```python
from build123d import *

# Parameters (mm, degrees)
BOSS_EXTRUDE1_DEPTH = 19.05
SKETCH2_R           = 3.96875
CUT_EXTRUDE1_DEPTH  = 19.05
SKETCH3_W           = 457.2
SKETCH3_H           = 152.4
BOSS_EXTRUDE3_DEPTH = 19.05
SKETCH4_W           = 457.2
SKETCH4_H           = 152.4
CUT_EXTRUDE2_DEPTH  = 25.4
CUT_EXTRUDE3_DEPTH  = 25.4
BOSS_EXTRUDE4_DEPTH = 3.175


with BuildPart() as part:
    # Sketch1 → Boss-Extrude1 (new body)
    with BuildSketch(Plane(origin=(0, 0, 0), x_dir=(1, 0, 0), z_dir=(0, 1, 0))):
        Polygon((57.15, 19.05), (0, 19.05), (0, 0), (66.037825848, 0), (97.808358016, 38.1), (336.311308439, 38.1), (400.965853894, -12.7), (431.8, -12.7), (342.9, 57.15), (88.9, 57.15), align=None)
    extrude(amount=BOSS_EXTRUDE1_DEPTH)

    # Sketch2 → Cut-Extrude1 (cut)
    with BuildSketch(Plane.XY):
        with Locations((8.89, 9.525)):
            Circle(SKETCH2_R)
        with Locations((56.515, 9.525)):
            Circle(SKETCH2_R)
    extrude(amount=-CUT_EXTRUDE1_DEPTH, mode=Mode.SUBTRACT)

    # Sketch4 → Cut-Extrude2 (cut)
    with BuildSketch(Plane(origin=(0, 0, 0), x_dir=(1, 0, 0), z_dir=(0, 1, 0))):
        with Locations((215.9, 38.1)):
            Rectangle(SKETCH4_W, SKETCH4_H)
    extrude(amount=CUT_EXTRUDE2_DEPTH, mode=Mode.SUBTRACT)


with BuildPart() as body_2:
    # Sketch3 → Boss-Extrude3 (new body)
    with BuildSketch(Plane.XZ):
        with Locations((215.9, -38.1)):
            Rectangle(SKETCH3_W, SKETCH3_H)
        Polygon((400.965853894, 12.7), (431.8, 12.7), (342.9, -57.15), (88.9, -57.15), (57.15, -19.05), (0, -19.05), (0, 0), (66.037825848, 0), (97.808358016, -38.1), (336.311308439, -38.1), align=None, mode=Mode.SUBTRACT)
    extrude(amount=BOSS_EXTRUDE3_DEPTH)

    # Sketch5 → Cut-Extrude3 (cut)
    with BuildSketch(Plane.XZ.offset(19.05)):
        Polygon((57.15, -19.05), (0, -19.05), (-12.7, -19.05), (-12.7, -114.3), (444.5, -114.3), (444.5, 38.1), (431.8, 38.1), (431.8, 12.7), (342.9, -57.15), (88.9, -57.15), align=None)
    extrude(amount=-CUT_EXTRUDE3_DEPTH, mode=Mode.SUBTRACT)

    # Sketch6 → Boss-Extrude4 (add)
    with BuildSketch(Plane.XZ.offset(19.05)):
        Polygon((400.965853894, 12.7), (336.311308439, -38.1), (336.311308439, -57.15), (431.8, -57.15), (431.8, 12.7), align=None)
        Polygon((336.311308439, -57.15), (336.311308439, -38.1), (97.808358016, -38.1), (66.037825848, 0), (0, 0), (0, -19.05), (-12.7, -19.05), (-12.7, -57.15), align=None)
        Polygon((97.808358016, -38.1), (336.311308439, -38.1), (336.311308439, 38.1), (-12.7, 38.1), (-12.7, -19.05), (0, -19.05), (0, 0), (66.037825848, 0), align=None)
        Polygon((336.311308439, 38.1), (336.311308439, -38.1), (400.965853894, 12.7), (431.8, 12.7), (431.8, 38.1), align=None)
    extrude(amount=BOSS_EXTRUDE4_DEPTH)


solid = body_2.part
```
For this review, take the finished solid that the model builds, in its own axes (mm). A direction names the side the tool comes from. Coordinates: 2 decimals unless noted, no trailing zeros. Write each loop counter-clockwise with the first axis right and the second up, starting at its lowest first coordinate (ties: lowest second). Pieces come first, ordered by that corner, then holes.
(1) Add section B-B on x = 27. Give the boundary of the cut face in (y, z) (3 decimals).
(2) Add section C-C on z = -29. Give the boundary of the cut face in (x, y) (3 decimals).
(3) Add section A-A on y = -7.5. Give the boundary of the cut face in (x, z).
(4) Tool access review of faces 1 (the face through (-6, -10, -19.05)), 2 (the face through (33, -9, 0)), 3 (the face through (368.186, -9.392, -13.056)): name each direction out of +Z, -Z, +X, -X, +Y, -Y from which nothing blocks a thin tool from reaching the whole face with its end or side.
(5) Add section D-D on x = 104.5. Give the boundary of the cut face in (y, z) (3 decimals), then the cut area to 3 significant figures.
(6) The part is to be moulded in two halves that separate along X. For faces 4 (the face through (431.8, -14, 15)), 5 (the face through (0, -9, -10)), 6 (the face through (206, 0, 9)), say which applies: +X half, -X half, draft (parallel to the pull), parting line (faces both ways), or undercut.
(7) Wall thickness on probe 1 along Y at (x, z) = (406, -5) (3 decimals); probe 2 along Z at (x, y) = (120.5, -14.75); probe 3 along Z at (x, y) = (6, -15.75): over which ranges is each line inside the solid? List them lowest first.
(8) For pin 1 Ø5.5 at (x, y) = (24.5, -5.5) entering from -Z; pin 2 Ø10 at (x, y) = (-4, -14) entering from -Z; pin 3 Ø6 at (x, y) = (229, -3.5) entering from -Z, all flat-tipped, find the tip position at first contact; note any pin that passes through.
Answer sheet:
1. outline: (-22.225, -57.15) - (-19.05, -57.15) - (-19.05, 0) - (0, 0) - (0, 38.1) - (-22.225, 38.1) - close
2. outline: (-12.7, -22.225) - (431.8, -22.225) - (431.8, -19.05) - (347.893, -19.05) - (347.893, 0) - (90.22, 0) - (90.22, -19.05) - (-12.7, -19.05) - close
3. outline: (-12.7, -19.05) - (0, -19.05) - (0, 0) - (66.04, 0) - (97.81, -38.1) - (336.31, -38.1) - (400.97, 12.7) - (431.8, 12.7) - (431.8, 38.1) - (-12.7, 38.1) - close
4. face 1: -Z, -X, +Y
4. face 2: -Z, +Y
4. face 3: -Z, +X, +Y
5. outline: (-22.225, -57.15) - (-19.05, -57.15) - (-19.05, -38.1) - (0, -38.1) - (0, 38.1) - (-22.225, 38.1) - close
5. area: 1,750 mm2
6. face 4: +X half
6. face 5: undercut
6. face 6: draft
7. probe 1: y = -22.225 to -19.05
7. probe 2: z = -38.1 to 38.1
7. probe 3: z = 0 to 38.1
8. pin 1: stops at z = 0
8. pin 2: stops at z = -19.05
8. pin 3: stops at z = -38.1
